Source: CAD feature listing. Evaluate the final solid. Frame: model axes, mm. A direction names the side the tool comes from. Coordinates: 2 decimals unless noted, no trailing zeros. Order: outer loops, then holes, each group sorted by start corner. A loop starts at its lowest first (then second) coordinate and runs counter-clockwise, first axis right, second up. Notation, with made-up numbers: (47, -36.5) - (70, -36.5) arc R35 ccw to (70, -4.5) - close; hole circle Ø5 at (81, 68.5). An arc over 180 degrees is marked (long way). One line per question, with ' | ' between items.
from build123d import *

# Parameters (mm, degrees)
SKETCH1_W           = 120
SKETCH1_H           = 50
SKETCH1_R           = 5
BOSS_EXTRUDE4_DEPTH = 10
SKETCH1_6_R         = 6
SKETCH1_6_R_2       = 10
SKETCH1_6_R_3       = 3
BOSS_EXTRUDE5_DEPTH = 32
CUT_EXTRUDE1_START  = 2
SKETCH1_9_R         = 3
CUT_EXTRUDE1_DEPTH  = 32
CUT_EXTRUDE2_START  = 32
SKETCH1_10_R        = 6
CUT_EXTRUDE2_DEPTH  = 5
CHAMFER1_SIZE       = 5


with BuildPart() as part:
    # Sketch1 → Boss-Extrude4 (new body)
    with BuildSketch(Plane(origin=(0, 0, 0), x_dir=(1, 0, 0), z_dir=(0, 1, 0))):
        Rectangle(SKETCH1_W, SKETCH1_H)
        with Locations(Location((50, -15, 0), (0, 0, 270))):
            Circle(SKETCH1_R, mode=Mode.SUBTRACT)
        with Locations(Location((50, 15, 0), (0, 0, 270))):
            Circle(SKETCH1_R, mode=Mode.SUBTRACT)
        with Locations(Location((-50, -15, 0), (0, 0, 270))):
            Circle(SKETCH1_R, mode=Mode.SUBTRACT)
        with Locations(Location((-50, 15, 0), (0, 0, 270))):
            Circle(SKETCH1_R, mode=Mode.SUBTRACT)
        Polygon((-8.3, -20), (-20, -8.3), (-35, -8.3), (-35, 8.3), (-20, 8.3), (-8.3, 20), (8.3, 20), (20, 8.3), (35, 8.3), (35, -8.3), (20, -8.3), (8.3, -20), align=None, mode=Mode.SUBTRACT)
    extrude(amount=BOSS_EXTRUDE4_DEPTH)

    # Sketch1<6> → Boss-Extrude5 (add)
    # profile 1 of 5: a face of its own
    with BuildSketch(Plane(origin=(0, 0, 0), x_dir=(1, 0, 0), z_dir=(0, 1, 0))):
        Polygon((-20, -8.3), (-35, -8.3), (-35, 8.3), (-20, 8.3), (-8.3, 20), (8.3, 20), (20, 8.3), (35, 8.3), (35, -8.3), (20, -8.3), (8.3, -20), (-8.3, -20), align=None)
        with Locations((26, 0)):
            Circle(SKETCH1_6_R, mode=Mode.SUBTRACT)
        with Locations((-26, 0)):
            Circle(SKETCH1_6_R, mode=Mode.SUBTRACT)
        with Locations(Location((0, 0, 0), (0, 0, 270))):
            Circle(SKETCH1_6_R_2, mode=Mode.SUBTRACT)
    # profile 2 of 5: a face of its own
    with BuildSketch(Plane(origin=(0, 0, 0), x_dir=(1, 0, 0), z_dir=(0, 1, 0))):
        with Locations((-26, 0)):
            Circle(SKETCH1_6_R)
        with Locations((-26, 0)):
            Circle(SKETCH1_6_R_3, mode=Mode.SUBTRACT)
    # profile 3 of 5: a face of its own
    with BuildSketch(Plane(origin=(0, 0, 0), x_dir=(1, 0, 0), z_dir=(0, 1, 0))):
        with Locations((-26, 0)):
            Circle(SKETCH1_6_R_3)
    # profile 4 of 5: a face of its own
    with BuildSketch(Plane(origin=(0, 0, 0), x_dir=(1, 0, 0), z_dir=(0, 1, 0))):
        with Locations((26, 0)):
            Circle(SKETCH1_6_R)
        with Locations((26, 0)):
            Circle(SKETCH1_6_R_3, mode=Mode.SUBTRACT)
    # profile 5 of 5: a face of its own
    with BuildSketch(Plane(origin=(0, 0, 0), x_dir=(1, 0, 0), z_dir=(0, 1, 0))):
        with Locations((26, 0)):
            Circle(SKETCH1_6_R_3)
    extrude(amount=BOSS_EXTRUDE5_DEPTH)

    # Sketch1<9> → Cut-Extrude1 (cut)
    with BuildSketch(Plane(origin=(0, 0, 0), x_dir=(1, 0, 0), z_dir=(0, 1, 0)).offset(CUT_EXTRUDE1_START)):
        with Locations(Location((-26, 0, 0), (0, 0, 270))):
            Circle(SKETCH1_9_R)
        with Locations(Location((26, 0, 0), (0, 0, 270))):
            Circle(SKETCH1_9_R)
    extrude(amount=CUT_EXTRUDE1_DEPTH, mode=Mode.SUBTRACT)

    # Sketch1<10> → Cut-Extrude2 (cut)
    with BuildSketch(Plane(origin=(0, 0, 0), x_dir=(1, 0, 0), z_dir=(0, 1, 0)).offset(CUT_EXTRUDE2_START)):
        with Locations(Location((-26, 0, 0), (0, 0, 270))):
            Circle(SKETCH1_10_R)
        with Locations(Location((26, 0, 0), (0, 0, 270))):
            Circle(SKETCH1_10_R)
    extrude(amount=-CUT_EXTRUDE2_DEPTH, mode=Mode.SUBTRACT)

    # Chamfer1
    chamfer1_edges = [part.edges().sort_by_distance(p)[0] for p in [
        (60, 5, 25),
        (-60, 5, 25),
        (-60, 5, -25),
        (60, 5, -25),
    ]]
    chamfer(chamfer1_edges, length=CHAMFER1_SIZE)


solid = part.part
(1) Pin query (flat end, axial travel): P1, Ø5, axis at x = 34.5, y = 19.5, coming from the +Z side; P2, Ø7.5, axis at x = -25, y = 23, coming from the -Z side; P3, Ø3, axis at x = -39.5, z = -10.5, coming from the +Y side. Return the tip coordinate at first contact, or that it passes through.
Taken from the geometry:
P1: stops at z = 8.3 | P2: stops at z = -8.3 | P3: stops at y = 10
(2) Set-up query: faces 4 (the flat face through (-26, 2, 0)), 5 (the flat face through (14.2, 20.8, 14.1)), 6 (the flat face through (27, 21, -8.3)). Return all of +Z, -Z, +X, -X, +Y, -Y with unobstructed straight access to the full face (end or side cutting, diameter ignored); none if empty.
Taken from the geometry:
face 4: +Y | face 5: +Z, +X, +Y | face 6: -Z, +X, +Y
(3) Pull-direction query (X, two-part tool) for faces 1 (the flat face through (-14.1, 20.8, 14.2)), 2 (the flat face through (14.1, 20.8, -14.2)), 3 (the flat face through (25, 27, -3)); classes: pulls with the +X half, pulls with the -X half, needs draft (parallel to the pull), parting line crosses it, or undercut.
Taken from the geometry:
face 1: pulls with the -X half | face 2: pulls with the +X half | face 3: undercut
(4) Cut plane C-C (x = -50). Return the cut outline in (y, z).
Taken from the geometry:
outline: (0, -25) - (10, -25) - (10, -20) - (0, -20) - close; (0, -10) - (10, -10) - (10, 10) - (0, 10) - close; (0, 20) - (10, 20) - (10, 25) - (0, 25) - close
(5) Cut plane A-A (z = 0). Return the cut outline in (x, y), and give its area (3 significant figures).
Taken from the geometry:
outline: (-60, 0) - (-10, 0) - (-10, 32) - (-20, 32) - (-20, 27) - (-23, 27) - (-23, 2) - (-29, 2) - (-29, 27) - (-32, 27) - (-32, 32) - (-35, 32) - (-35, 10) - (-60, 10) - close; (10, 0) - (60, 0) - (60, 10) - (35, 10) - (35, 32) - (32, 32) - (32, 27) - (29, 27) - (29, 2) - (23, 2) - (23, 27) - (20, 27) - (20, 32) - (10, 32) - close | area: 1,680 mm²
(6) Cut plane B-B (y = 23). Return the cut outline in (x, z).
Taken from the geometry:
outline: (-35, -8.3) - (-20, -8.3) - (-8.3, -20) - (8.3, -20) - (20, -8.3) - (35, -8.3) - (35, 8.3) - (20, 8.3) - (8.3, 20) - (-8.3, 20) - (-20, 8.3) - (-35, 8.3) - close; hole circle Ø6 at (-26, 0); hole circle Ø20 at (0, 0); hole circle Ø6 at (26, 0)
(7) Cut plane D-D (z = 15). Return the cut outline in (x, y), and give its area (3 significant figures).
Taken from the geometry:
outline: (-60, 0) - (-55, 0) - (-55, 10) - (-60, 10) - close; (-45, 0) - (45, 0) - (45, 10) - (13.3, 10) - (13.3, 32) - (-13.3, 32) - (-13.3, 10) - (-45, 10) - close; (55, 0) - (60, 0) - (60, 10) - (55, 10) - close | area: 1,590 mm²
(8) Material intervals for L1, parallel to X at y = 28.75, z = 0; L2, parallel to Z at x = -54, y = 3; L3, parallel to X at y = 6, z = -15, sorted ascending. Write a range as from..to.
Taken from the geometry:
L1: x = -35..-32, -20..-10, 10..20, 32..35 | L2: z = -25..-18, -12..12, 18..25 | L3: x = -60..-55, -45..45, 55..60
